```python
from build123d import *

# Parameters (mm, degrees)
F0_W      = 24.785
F0_H      = 24.785
F0_R      = 4.2045
F1_DEPTH  = 5.6
F1_FACE_W = 24.785
F1_FACE_H = 24.785
F1_FACE_R = 4.2045
F2_DEPTH  = 1.6


with BuildPart() as f1:
    # F0 (on Top) → F1 (new body)
    with BuildSketch(Plane.XY):
        with Locations((-39.635155, 26.570821)):
            Rectangle(F0_W, F0_H)
        with Locations((-39.635155, 26.570821)):
            Circle(F0_R, mode=Mode.SUBTRACT)
    extrude(amount=F1_DEPTH)

    # F1_face (on face) → F2 (join)
    with BuildSketch(Plane(origin=(-39.635155, 26.570821, 5.6), x_dir=(1, 0, 0), z_dir=(0, 0, 1))):
        Rectangle(F1_FACE_W, F1_FACE_H)
        Circle(F1_FACE_R, mode=Mode.SUBTRACT)
    extrude(amount=-F2_DEPTH)


solid = f1.part
```
Verification items for the finished model (mm, model axes). Round coordinates to 2 decimals unless told otherwise and drop trailing zeros. Loops run counter-clockwise (first coordinate to the right, second up) from the corner with the lowest first, then second, coordinate; pieces in that order, holes last. Notation, with made-up numbers: (66.25, 4) -> (100.25, 4) arc R31 cw to (100.25, 35) -> close; hole circle Ø8 at (79.25, 39). An arc over 180 degrees is marked (long way). Answer as a JSON object with one key per item and string values.
Q1. Section check C-C (z = 5.1). Record the boundary of the cut face in (x, y), then the cut area to 3 significant figures.
Data:
{"outline": "(-52.03, 14.18) -> (-27.24, 14.18) -> (-27.24, 38.96) -> (-52.03, 38.96) -> close; hole circle Ø8.41 at (-39.64, 26.57)", "area": "559 mm2"}
Q2. Draft check along Y on faces 1 (the flat face through (-34, 27, 5.6)), 2 (the flat face through (-40, 38.963, 3)), 3 (the cylindrical face through (-43.836, 26.756, 2.761)). Enter one of: pulls with the +Y half, pulls with the -Y half, needs draft (parallel to the pull), parting line crosses it, or undercut.
Data:
{"face 1": "needs draft", "face 2": "pulls with the +Y half", "face 3": "undercut"}
Q3. Scan lines: line 1 (Y direction, x = -39.75, z = 2.6); line 2 (X direction, y = 27.25, z = 4.4); line 3 (Y direction, x = -36.5, z = 0.55). Record each from-to range of solid material in increasing order. Write a range as from..to.
Data:
{"line 1": "y = 14.18..22.37, 30.77..38.96", "line 2": "x = -52.03..-43.78, -35.49..-27.24", "line 3": "y = 14.18..23.77, 29.37..38.96"}
Q4. Section check A-A (x = -40.5). Record the boundary of the cut face in (y, z).
Data:
{"outline": "(14.18, 0) -> (22.46, 0) -> (22.46, 5.6) -> (14.18, 5.6) -> close; (30.69, 0) -> (38.96, 0) -> (38.96, 5.6) -> (30.69, 5.6) -> close"}
Q5. Section check B-B (x = -43.5). Record the boundary of the cut face in (y, z), then the cut area to 3 significant figures.
Data:
{"outline": "(14.18, 0) -> (24.92, 0) -> (24.92, 5.6) -> (14.18, 5.6) -> close; (28.23, 0) -> (38.96, 0) -> (38.96, 5.6) -> (28.23, 5.6) -> close", "area": "120 mm2"}
